Here's the drawing with two shaded views (mm, measured from the low corner). I have some questions. Coordinates: 2 decimals unless noted, no trailing zeros. Write each loop counter-clockwise with the first axis right and the second up, starting at its lowest first coordinate (ties: lowest second). Pieces come first, ordered by that corner, then holes.
Item 1: I want a section at B-B on x = 45. Please give me the cut outline in (y, z).
Item 2: I want a section at D-D on x = 15. Please give me the cut outline in (y, z).
Item 3: For P1, Ø0.6, axis at y = 1, z = 155.5, coming from the -X side, with a flat end and sliding along its axis, tell me the tip position at first contact or that it passes through.
Item 4: If I drill on probe 1 along Z at (x, y) = (203.76, 0.55); probe 2 along X at (y, z) = (0.75, 60.5); probe 3 along Z at (x, y) = (14, 1.35), over which ranges is the centre line in solid material (lowest first)?
Item 5: I want a section at A-A on z = 60.5. Please give me the cut outline in (x, y), then the cut area to 3 significant figures.
Item 6: I want a section at C-C on y = 0.6. Please give me the cut outline in (x, z), then the cut area to 3 significant figures.
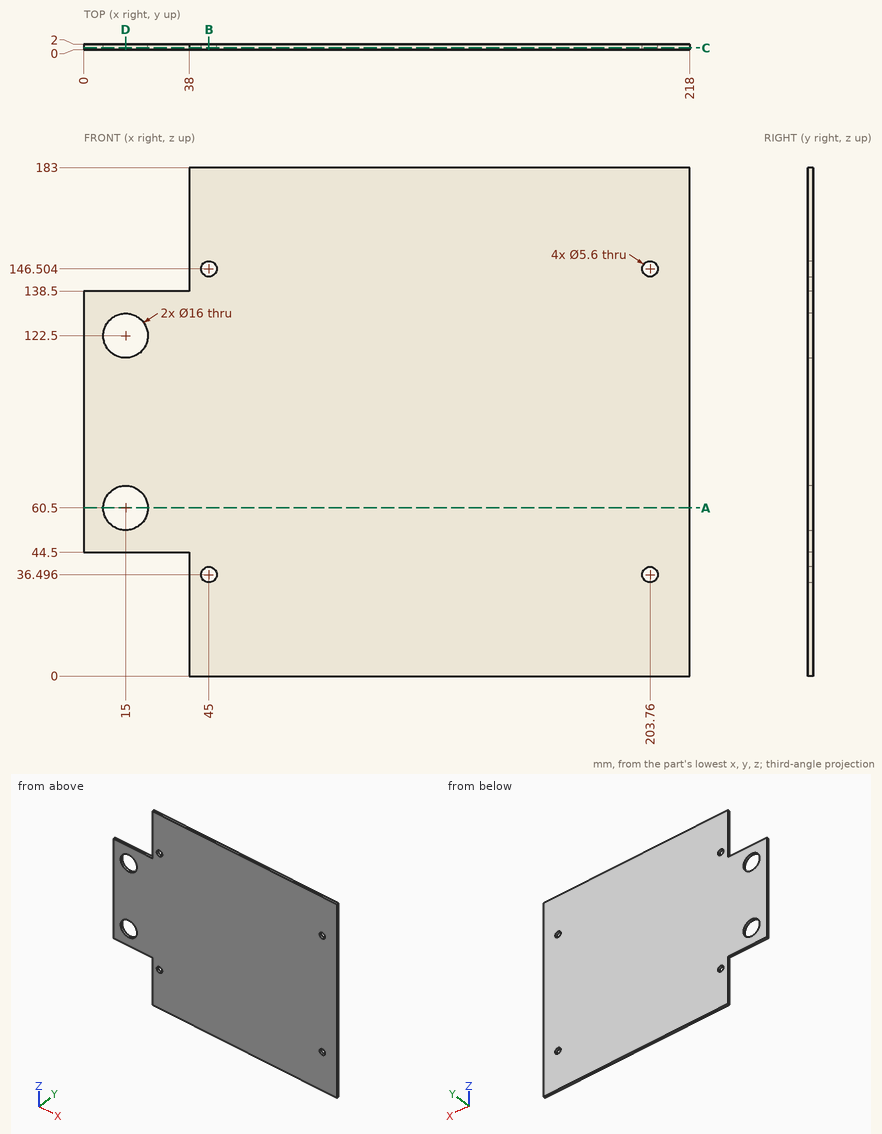
Response values:
1. outline: (0, 0) - (2, 0) - (2, 33.7) - (0, 33.7) - close; (0, 39.3) - (2, 39.3) - (2, 143.7) - (0, 143.7) - close; (0, 149.3) - (2, 149.3) - (2, 183) - (0, 183) - close
2. outline: (0, 44.5) - (2, 44.5) - (2, 52.5) - (0, 52.5) - close; (0, 68.5) - (2, 68.5) - (2, 114.5) - (0, 114.5) - close; (0, 130.5) - (2, 130.5) - (2, 138.5) - (0, 138.5) - close
3. P1: stops at x = 38
4. probe 1: z = 0 to 33.7, 39.3 to 143.7, 149.3 to 183
4. probe 2: x = 0 to 7, 23 to 218
4. probe 3: z = 44.5 to 52.56, 68.44 to 114.56, 130.44 to 138.5
5. outline: (0, 0) - (7, 0) - (7, 2) - (0, 2) - close; (23, 0) - (218, 0) - (218, 2) - (23, 2) - close
5. area: 404 mm2
6. outline: (0, 44.5) - (38, 44.5) - (38, 0) - (218, 0) - (218, 183) - (38, 183) - (38, 138.5) - (0, 138.5) - close; hole circle Ø16 at (15, 60.5); hole circle Ø16 at (15, 122.5); hole circle Ø5.6 at (45, 36.5); hole circle Ø5.6 at (45, 146.5); hole circle Ø5.6 at (203.76, 36.5); hole circle Ø5.6 at (203.76, 146.5)
6. area: 36,000 mm2
